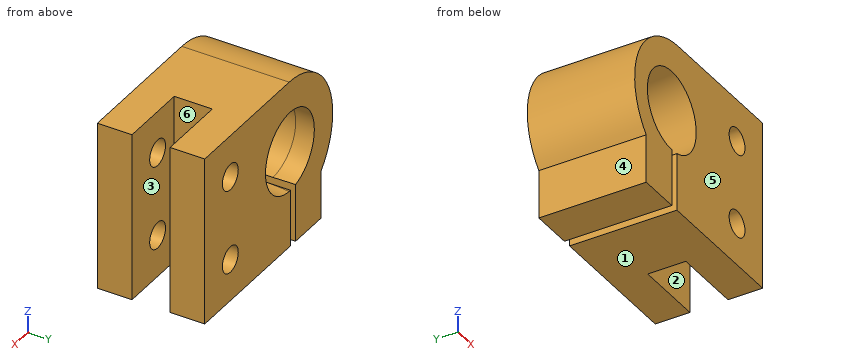
Autodesk Inventor part; units mm, degrees
ref_plane "YZ Plane" through (0, 0, 0) normal (1, 0, 0) x (0, 1, 0)
ref_plane "XZ Plane" through (0, 0, 0) normal (0, 1, 0) x (-1, 0, 0)
ref_plane "XY Plane" through (0, 0, 0) normal (0, 0, 1) x (1, 0, 0)
sketch "Sketch1" plane through (0, 0, 0) normal (0, 1, 0) x (-1, 0, 0)
  line L0 (50, 0) -> (50, 40)
  line L1 (50, 40) -> (0, 40)
  line L2 (0, 40) -> (0, 0)
  line L3 (0, 0) -> (10, 0)
  line L4 (10, 0) -> (10, 10)
  line L5 (10, 10) -> (10, 30)
  circle A0 centre (10, 30) radius 3.1
  circle A1 centre (10, 10) radius 3.1
  line L6 (45.5, 0) -> (45.5, 11.4783)
  line L7 (0, 0) -> (33.5, 0)
  line L8 (35.5, 0) -> (35.5, 18.6699)
  line L9 (50, 40) -> (45.5, 40)
  line L10 (45.5, 40) -> (45.5, 35.5)
  line L11 (45.5, 35.5) -> (45.5, 34.5217)
  line L12 (45.5, 23) -> (33, 23)
  arc A2 (45.5, 11.4783) -> (33, 40) centre (33, 23) ccw
  line L13 (0, 0) -> (33.5, 0)
  line L14 (35.5, 0) -> (45.5, 0)
  line L15 (33.5, 0) -> (33.5, 18.0251)
  line L16 (0, 0) -> (33.5, 0)
  line L17 (35.5, 0) -> (45.5, 0)
  line L18 (33, 23) -> (28, 23)
  line L19 (33, 23) -> (38, 23)
  arc A3 (35.5, 18.6699) -> (38, 23) centre (33, 23) ccw
  arc A4 (28, 23) -> (33.5, 18.0251) centre (33, 23) ccw
  dimension "d0" = 50
  dimension "d1" = 40
  dimension "d2" = 10
  dimension "d3" = 10
  dimension "d4" = 20
  dimension "d5" = 6.2
  dimension "d6" = 6.2
  dimension "d7" = 45.5
  dimension "d8" = 35.5
  dimension "d9" = 4.5
  dimension "d10" = 4.5
  dimension "d13" = 12.5
  dimension "d14" = 12.5
  dimension "d15" = 2
extrude "Extrusion1" add sketch "Sketch1" along normal blind 25.4 contours A2 L6 L14 L8 A3 L12 L18 A4 L15 L7 L3 L2 L1
sketch "Sketch2" plane through (-33, 0, 40) normal (0, 0, 1) x (1, 0, 0)
  line L0 (33, 0) -> (33, 8.2)
  line L1 (33, 0) -> (33, 25.4)
  line L2 (33, 8.2) -> (16.5, 8.2)
  line L3 (16.5, 8.2) -> (16.5, 17.2)
  line L4 (16.5, 17.2) -> (33, 17.2)
  line L5 (33, 17.2) -> (33, 8.2)
  dimension "d18" = 8.2
  dimension "d19" = 16.5
  dimension "d20" = 9
extrude "Extrusion2" cut sketch "Sketch2" against normal through all
sketch "Sketch6" plane through (-28, 0, 23) normal (0, 0, -1) x (-1, 0, 0)
  line L0 (10, 25.4) -> (5.5, 25.4)
  line L1 (0, 25.4) -> (5.5, 25.4)
  line L2 (5.5, 25.4) -> (7.7222, 0)
  line L3 (7.5, 0) -> (17.5, 0)
  line L4 (5.5, 25.4) -> (30.997, 25.4) construction
  line L5 (7.5, 0) -> (8.3716, -9.9619)
  line L6 (7.5, 0) -> (17.5, 0) construction
  line L7 (15.2207, 20.7519) -> (-3.707, 19.0959)
  line L8 (-3.707, 19.0959) -> (-1.0923, -10.7899)
  line L9 (-1.0923, -10.7899) -> (8.3716, -9.9619)
  line L10 (8.3716, -9.9619) -> (5.7569, 19.9239)
  line L11 (8.3716, -9.9619) -> (38.3716, -9.9619) construction
  line L12 (8.3716, -9.9619) -> (5.7569, 19.9239)
  line L13 (-1.0923, -10.7899) -> (-3.707, 19.0959)
  line L14 (-1.0923, -10.7899) -> (28.9077, -10.7899) construction
  line L15 (-3.707, 19.0959) -> (5.7569, 19.9239)
  line L16 (5.7569, 19.9239) -> (8.3716, -9.9619)
  point P0 (-28, 0)
  dimension "d35" = 85
  dimension "d36" = 10
  dimension "d37" = 85
  dimension "d43" = 30
  dimension "d44" = 90
  dimension "d45" = 30
  dimension "d47" = 30
  dimension "d48" = 95
  dimension "d49" = 9.5
revolve "Revolution2" cut sketch "Sketch6" angle 360 about axis through (-36.3716, -9.9619, 23) along (0.0871557, 0.9961947, 0) contours L10 L5 L9 L8 L7
sketch "Sketch7" plane through (-35.5, 20.0764, 13.6625) normal (-0.0871557, -0.9961947, 0) x (0.9961947, -0.0871557, 0)
  arc A0 (2.0076, -0.159) -> (0, 0) centre (1.7498, 9.3375) ccw
  circle A1 centre (1.7498, 9.3375) radius 9.5
  point P0 (37.1147, -13.6625)
extrude "Extrusion3" cut sketch "Sketch7" against normal blind 10
properties part number "suporte-eixo"
Input: part model. Units: mm. Frame: model coordinates. Face numbers are marked on the shaded views. A direction names the side the tool comes from. Coordinates: 2 decimals unless noted, no trailing zeros. Loops run counter-clockwise (first coordinate to the right, second up) from the corner with the lowest first, then second, coordinate; pieces in that order, holes last. Notation, with made-up numbers: M 47,81 L 74,81 A20 cw 74,89 Z; hole C -38,20.5 d10. An arc over 180 degrees is marked long. Use a Markdown table: item, result. Add a question column.
1) Line query: L1, parallel to Z at x = -10, y = 19; L2, parallel to X at y = 11.5, z = 2; L3, parallel to X at y = 23, z = 10. Output: solid intervals per line, ascending. Write a range as from..to.
2) Section C-C, the plane z = 22. Return the cut outline in (x, y).
3) Draft query along Y for the marked faces 3, 4, 5 and 6. Return one class per face: +Y half, -Y half, draft (parallel to the pull), parting line (faces both ways), or undercut.
4) Pin query (flat end, axial travel): P1, Ø12.5, axis at y = 15.5, z = 3, coming from the -X side; P2, Ø10, axis at y = 8, z = 30, coming from the -X side; P3, Ø7, axis at y = 9, z = 10, coming from the -X side; P4, Ø3.5, axis at x = -10, z = 30, coming from the -Y side. Return the tip coordinate at first contact, or that it passes through.
5) Section B-B, the plane z = 10. Return the cut outline in (x, y).
6) Section D-D, the plane z = 30. Return the cut outline in (x, y).
7) Set-up query: the marked faces 1 and 2. Return all of +Z, -Z, +X, -X, +Y, -Y with unobstructed straight access to the full face (end or side cutting, diameter ignored); none if empty.
8) Section A-A, the plane x = -10. Return the cut outline in (y, z).
Answer below:
| question | item | result |
|---|---|---|
| 1 | L1 | 0..6.9, 13.1..26.9, 33.1..40 |
| 1 | L2 | -45.5..-35.5, -33.5..-16.5 |
| 1 | L3 | -45.5..-35.5, -33.5..-13.1, -6.9..0 |
| 2 | outline | M -49.97,0 L -44.98,0 L -43.17,20.75 L -42.76,25.4 L -49.97,25.4 Z; M -26.02,0 L 0,0 L 0,8.2 L -16.5,8.2 L -16.5,17.2 L 0,17.2 L 0,25.4 L -23.79,25.4 L -24.35,19.1 Z |
| 3 | face 3 | undercut |
| 3 | face 4 | draft |
| 3 | face 5 | -Y half |
| 3 | face 6 | undercut |
| 4 | P1 | x = -45.5 |
| 4 | P2 | x = -49.88 |
| 4 | P3 | x = -47.1 |
| 4 | P4 | through |
| 5 | outline | M -45.5,0 L -35.5,0 L -35.5,25.4 L -45.5,25.4 Z; M -33.5,0 L -13.1,0 L -13.1,8.2 L -16.5,8.2 L -16.5,17.2 L -13.1,17.2 L -13.1,25.4 L -33.5,25.4 Z; M -6.9,0 L 0,0 L 0,8.2 L -6.9,8.2 Z; M -6.9,17.2 L 0,17.2 L 0,25.4 L -6.9,25.4 Z |
| 6 | outline | M -48.49,0 L -41.95,0 L -40.16,20.48 L -39.73,25.4 L -48.49,25.4 Z; M -29.05,0 L -13.1,0 L -13.1,8.2 L -16.5,8.2 L -16.5,17.2 L -13.1,17.2 L -13.1,25.4 L -26.83,25.4 L -27.36,19.36 Z; M -6.9,0 L 0,0 L 0,8.2 L -6.9,8.2 Z; M -6.9,17.2 L 0,17.2 L 0,25.4 L -6.9,25.4 Z |
| 7 | face 1 | -Z, +X, -X, +Y, -Y |
| 7 | face 2 | +Z, -Z, +X |
| 8 | outline | M 0,0 L 8.2,0 L 8.2,6.9 L 0,6.9 Z; M 0,13.1 L 8.2,13.1 L 8.2,26.9 L 0,26.9 Z; M 0,33.1 L 8.2,33.1 L 8.2,40 L 0,40 Z; M 17.2,0 L 25.4,0 L 25.4,6.9 L 17.2,6.9 Z; M 17.2,13.1 L 25.4,13.1 L 25.4,26.9 L 17.2,26.9 Z; M 17.2,33.1 L 25.4,33.1 L 25.4,40 L 17.2,40 Z |
